```python
from build123d import *

# Parameters (mm, degrees)
SKETCH1_R           = 35
BOSS_EXTRUDE1_DEPTH = 9.5
SKETCH2_R           = 4
BOSS_EXTRUDE2_DEPTH = 15
SKETCH3_R           = 36.5
BOSS_EXTRUDE3_DEPTH = 2
SKETCH4_R           = 2.5
CUT_EXTRUDE1_DEPTH  = 17.5
SKETCH5_R           = 20
CUT_EXTRUDE2_DEPTH  = 7.5
CHAMFER1_SIZE       = 2.5


with BuildPart() as part:
    # Sketch1 → Boss-Extrude1 (new body)
    with BuildSketch(Plane(origin=(0, 0, 0), x_dir=(0, 0, -1), z_dir=(1, 0, 0))):
        Circle(SKETCH1_R)
    extrude(amount=BOSS_EXTRUDE1_DEPTH)

    # Sketch2 → Boss-Extrude2 (add)
    with BuildSketch(Plane(origin=(9.5, 0, 0), x_dir=(0, 0, -1), z_dir=(1, 0, 0))):
        Circle(SKETCH2_R)
    extrude(amount=BOSS_EXTRUDE2_DEPTH)

    # Sketch3 → Boss-Extrude3 (add)
    with BuildSketch(Plane.ZY.offset(-9.5)):
        Circle(SKETCH3_R)
    extrude(amount=BOSS_EXTRUDE3_DEPTH)

    # Sketch4 → Cut-Extrude1 (cut)
    with BuildSketch(Plane.ZY):
        with Locations((0, 27.5)):
            Circle(SKETCH4_R)
        with Locations((23.815698604, 13.75)):
            Circle(SKETCH4_R)
        with Locations((23.815698604, -13.75)):
            Circle(SKETCH4_R)
        with Locations((0, -27.5)):
            Circle(SKETCH4_R)
        with Locations((-23.815698604, -13.75)):
            Circle(SKETCH4_R)
        with Locations((-23.815698604, 13.75)):
            Circle(SKETCH4_R)
    extrude(amount=-CUT_EXTRUDE1_DEPTH, mode=Mode.SUBTRACT)

    # Sketch5 → Cut-Extrude2 (cut)
    with BuildSketch(Plane.ZY):
        Circle(SKETCH5_R)
    extrude(amount=-CUT_EXTRUDE2_DEPTH, mode=Mode.SUBTRACT)

    # Chamfer1
    chamfer1_edges = [part.edges().sort_by_distance(p)[0] for p in [
        (0, 0, 35),
        (0, 0, -20),
        (7.5, 0, -20),
    ]]
    chamfer(chamfer1_edges, length=CHAMFER1_SIZE)


solid = part.part
```
Source: CAD feature listing. Evaluate the final solid. Frame: model axes, mm. A direction names the side the tool comes from. Give positions to 0.01 mm unless a question says otherwise; leave off trailing zeros. Order: outer loops, then holes, each group sorted by start corner. A loop starts at its lowest first (then second) coordinate and runs counter-clockwise, first axis right, second up. Notation, with made-up numbers: (-17.75, 81) -> (12.25, 81) arc R24 cw to (12.25, 97) -> close; hole circle Ø11 at (77.25, 82.5). An arc over 180 degrees is marked (long way). Use a Markdown table: item, result.
Q1. First-contact query: P1, Ø8, axis at y = -8.5, z = -28, coming from the +X side; P2, Ø4, axis at x = 6.5, z = -8.5, coming from the +Y side; P3, Ø2, axis at x = 12, y = -5.5, coming from the -Z side; P4, Ø10.5, axis at y = -6, z = -2.5, coming from the -X side. Flat tips, straight axial feed; report the tip coordinate or a pass-through.
A:
| item | result |
|---|---|
| P1 | x = 9.5 |
| P2 | y = 35.87 |
| P3 | through |
| P4 | x = 7.5 |
Q2. Section A-A (z = 0). State how many separate pieces and enclosed holes the cut face has, and give its area (3 significant figures).
A:
| item | result |
|---|---|
| separate pieces | 3 |
| enclosed holes | 0 |
| area | 390 mm^2 |
Q3. Access query for faces 5 (the face through (16.895, -3.905, 0.867)), 6 (the face through (5, -21, 28)), 7 (the face through (24.5, 0, 0)). Directions: +Z, -Z, +X, -X, +Y, -Y. A direction counts if a zero-diameter tool reaches every point of the face in a straight line with its end or side. Return the directions, or none.
A:
| item | result |
|---|---|
| face 5 | +X |
| face 6 | -X |
| face 7 | +Z, -Z, +X, +Y, -Y |
Q4. Pull-direction query (Y, two-part tool) for faces 1 (the face through (8.514, -35.632, -7.912)), 2 (the face through (3.732, -19.524, -4.336)), 3 (the face through (7.5, -30, 19)), 4 (the face through (2.38, -17.85, 9.28)); classes: +Y half, -Y half, draft (parallel to the pull), parting line (faces both ways), or undercut.
A:
| item | result |
|---|---|
| face 1 | parting line |
| face 2 | undercut |
| face 3 | draft |
| face 4 | undercut |
Q5. Material intervals for line 1 (Y direction, x = 3.75, z = 0); line 2 (Y direction, x = 5, z = 25.5); line 3 (Z direction, x = 4.75, y = -12), sorted ascending. Write a range as [from, to].
A:
| item | result |
|---|---|
| line 1 | [-35, -30], [-25, -20], [20, 25], [30, 35] |
| line 2 | [-23.97, -15.6], [-11.9, 11.9], [15.6, 23.97] |
| line 3 | [-32.88, -25.6], [-22.03, -16], [16, 22.03], [25.6, 32.88] |
Q6. Section B-B (x = 21). Return the cut outline in (y, z), and give its area (3 significant figures).
A:
| item | result |
|---|---|
| outline | circle Ø8 at (0, 0) |
| area | 50.3 mm^2 |
